Read the model definition and answer for the solid it produces. Units are mm, in the model's axes. Face numbers are marked on the shaded views. A direction names the side the tool comes from. Round coordinates to 2 decimals unless told otherwise and drop trailing zeros. Write each loop counter-clockwise with the first axis right and the second up, starting at its lowest first coordinate (ties: lowest second). Pieces come first, ordered by that corner, then holes. Notation, with made-up numbers: (60.5, -9) - (103.5, -9) arc R12 cw to (103.5, 7) - close; hole circle Ø6 at (22, -17.5). An arc over 180 degrees is marked (long way). Use one line per item in the form item = value. Start each with the question number.
1) Consider line 1 along X through (y, z) = (-6.5, -2.75); line 2 along X through (y, z) = (-6.5, 2.9); line 3 along Z through (x, y) = (2.25, 1). Determine where each line is inside the solid, lowest interval first. Write a range as from..to.
2) The part is cut by section B-B, the plane z = 1.5. Count the separate pieces of the cut face and the enclosed holes in it, plus the area to 3 significant figures.
3) For the marked faces 4, 5 and 6, determine the directions among +Z, -Z, +X, -X, +Y, -Y from which every point of the face is accessible in a straight line to the end or side of a thin tool.
4) The part is cut by section A-A, the plane x = -2.75. Give the vertices of the cut face in (y, z), plus the area to 3 significant figures.
5) For a pull along X with two mould halves and no side action, classify the marked faces 1, 2 and 3 as released by +X, released by -X, zero draft, split by the parting line, or undercut.
6) Each of these flat-tipped pins is pushed along its axis until it touches: pin 1 (2 mm diameter, centred on x = -2.5, z = -5.5, fed in from +Y); pin 2 (6 mm diameter, centred on x = -3.5, y = 1.5, fed in from -Z); pin 3 (4.5 mm diameter, centred on x = -1, y = 5.5, fed in from -Z); pin 4 (1.2 mm diameter, centred on y = 0, z = 5.5, fed in from +X). Where does it stop, or does it pass through?
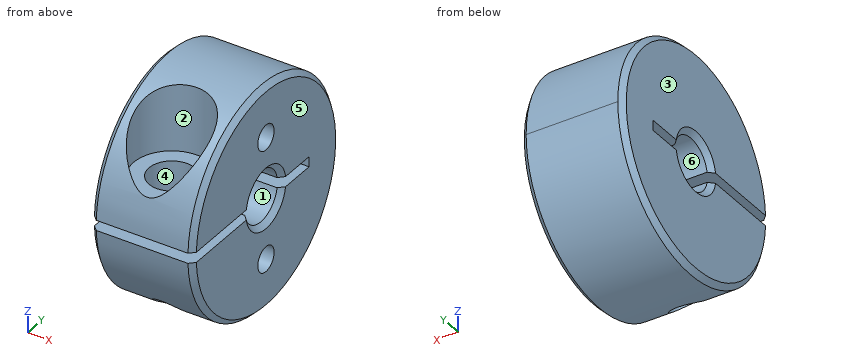
Autodesk Inventor part; units mm, degrees
ref_plane "body_screw_XY" through (0, -6.5, 4) normal (0, 0, 1) x (1, 0, 0)
ref_plane "body_screw_YZ" through (0, -6.5, 4) normal (1, 0, 0) x (0, 1, 0)
ref_plane "body_screw_ZX" through (0, -6.5, 4) normal (0, 1, 0) x (0, 0, 1)
sketch "Sketch_1" plane through (0, 0, 0) normal (0, 0, 1) x (1, 0, 0)
  line L0 (5, 0) -> (-5, 0)
  line L1 (-5, 10.5) -> (-5, 3)
  line L2 (-5, 3) -> (-4.5, 2.5)
  line L3 (-4.5, 2.5) -> (4.5, 2.5)
  line L4 (4.5, 2.5) -> (5, 3)
  line L5 (5, 3) -> (5, 10.5)
  line L6 (5, 10.5) -> (4.5, 11)
  line L7 (4.5, 11) -> (-4.5, 11)
  line L8 (-4.5, 11) -> (-5, 10.5)
revolve "Revolution1" add sketch "Sketch_1" angle 360 about axis through (5, 0, 0) along (1, 0, 0)
sketch "Sketch_2" plane through (0, 0, 0) normal (1, 0, 0) x (0, 1, 0)
  line L0 (-11, 0.5) -> (-11, -0.5)
  line L1 (-11, -0.5) -> (6.5, -0.5)
  line L2 (6.5, -0.5) -> (6.5, 0.5)
  line L3 (6.5, 0.5) -> (-11, 0.5)
extrude "Extrusion1" cut sketch "Sketch_2" along normal mid plane 10
sketch "Sketch_3" plane through (0, 0, 0) normal (1, 0, 0) x (0, 1, 0)
  line L0 (-6.5, 11) -> (-6.5, 0)
  line L1 (-6.5, 0) -> (-8.75, 0)
  line L2 (-8.75, 0) -> (-8.75, 4)
  line L3 (-8.75, 4) -> (-10.25, 4)
  line L4 (-10.25, 4) -> (-10.25, 11)
  line L5 (-10.25, 11) -> (-6.5, 11)
  line L6 (-6.5, 11) -> (-6.5, 0)
revolve "Revolution2" cut sketch "Sketch_3" angle 360 about axis through (0, -6.5, 11) along (0, 0, 1)
sketch "Sketch4" plane through (-4.5, -2.4495, -0.5) normal (0, 0, 1) x (1, 0, 0)
  point P0 (4.5, -4.0505)
hole "Hole1" at (0, -6.5, -0.5) direction (0, 0, -1) diameter 3.242 depth 9.75 countersink diameter 4 countersink angle 90
ref_plane "body_screw_XY" through (0, -6.5, 4) normal (0, 0, 1) x (1, 0, 0)
ref_plane "body_screw_YZ" through (0, -6.5, 4) normal (1, 0, 0) x (0, 1, 0)
ref_plane "body_screw_ZX" through (0, -6.5, 4) normal (0, 1, 0) x (0, 0, 1)
sketch "スケッチ5" plane through (5, 0, 0) normal (1, 0, 0) x (0, 0, -1)
  line L0 (0, 0) -> (-6, 0)
  point P0 (6, 0)
  dimension "d12" = 6
  dimension "d15" = 360
hole "穴2" at (5, 0, 6) at (5, 0, -6) direction (-1, 0, 0) diameter 2.459 depth 8.8
properties part number "SCS5-10b" material "鋼、炭素鋼"
Geometry results:
q1.line_1 = -5..-1.62, 1.62..5
q1.line_2 = -5..-2.25, 2.25..5
q1.line_3 = -10.95..-6.72, -5.28..-2.29, 2.29..5.28, 6.72..10.95
q2.separate_pieces = 2
q2.enclosed_holes = 1
q2.area = 161 mm2
q3.face_4 = +Z
q3.face_5 = +Z, -Z, +X, +Y, -Y
q3.face_6 = +X, -X
q4.outline = (-10.99, -0.5) arc R11 ccw (long way) to (-3.95, 10.27) - (-3.95, 4) - (-9.05, 4) - (-9.05, 6.25) arc R11 ccw to (-10.99, 0.5) - (-2.45, 0.5) arc R2.5 cw to (2.45, 0.5) - (6.5, 0.5) - (6.5, -0.5) - (2.45, -0.5) arc R2.5 cw to (-2.45, -0.5) - close; hole circle Ø2.46 at (0, -6); hole circle Ø2.46 at (0, 6)
q4.area = 315 mm2
q5.face_1 = zero draft
q5.face_2 = undercut
q5.face_3 = released by -X
q6.pin_1 = 10.04
q6.pin_2 = -11
q6.pin_3 = -10.51
q6.pin_4 = -3.8
